from build123d import *

# Parameters (mm, degrees)
F1_DEPTH    = 2.6
F0_W        = 3
F0_H        = 23.3
F0_W_2      = 4.4
F0_H_2      = 0.5
F0_W_3      = 3.9
F2_DEPTH    = 6.1
F3_T1_DEPTH = 6
F3_T3_DEPTH = 5.6650635095
F4_W        = 23
F4_H        = 2
F4_H_2      = 1.9
F5_DEPTH    = 2


# Not quite as in the source:
# - a fillet or chamfer that OpenCascade refuses, or shapes differently, is made with other operations: its cross-section is extruded or revolved along the edge and cut away or added


with BuildPart() as f1:
    # F0 (on Top) → F1 (new body)
    with BuildSketch(Plane.XY):
        Polygon((20, 0), (6.6, 0), (6.6, -5.35), (6.6, -5.85), (2.7, -5.85), (2.7, -5.35), (0, -5.35), (0, -21.3), (2.7, -21.3), (2.7, -20.8), (7.1, -20.8), (7.1, -21.3), (7.1, -23.3), (20, -23.3), align=None)
    extrude(amount=F1_DEPTH)

    # F0 (on Top) → F2 (join)
    with BuildSketch(Plane.XY):
        with Locations((21.5, -11.65)):
            Rectangle(F0_W, F0_H)
        Polygon((2.7, -21.3), (0, -21.3), (0, -23.3), (7.1, -23.3), (7.1, -21.3), align=None)
        Polygon((6.6, 0), (0, 0), (0, -5.35), (2.7, -5.35), (6.6, -5.35), align=None)
        with Locations((4.9, -21.05)):
            Rectangle(F0_W_2, F0_H_2)
        with Locations((4.65, -5.6)):
            Rectangle(F0_W_3, F0_H_2)
    extrude(amount=F2_DEPTH)

    # F3: fillet of radius 1 on 4 edges, made by hand

    # F3_s2 → F3_t1 (cut)
    with BuildSketch(Plane.XY.offset(2.6)):
        with BuildLine():
            ThreePointArc((7.1, -21.8), (6.8071067812, -21.0928932188), (6.1, -20.8))
            Line((6.1, -20.8), (7.1, -20.8))
            Line((7.1, -20.8), (7.1, -21.8))
        make_face()
        with BuildLine():
            ThreePointArc((5.6, -5.85), (6.3071067812, -5.5571067812), (6.6, -4.85))
            Line((6.6, -4.85), (6.6, -5.85))
            Line((6.6, -5.85), (5.6, -5.85))
        make_face()
    extrude(amount=F3_T1_DEPTH, mode=Mode.SUBTRACT)

    # F3_s4 → F3_t3 (cut)
    with BuildSketch(Plane.XY.offset(2.6)):
        with BuildLine():
            ThreePointArc((3.5660254038, -20.8), (3.0660254038, -20.9339745962), (2.7, -21.3))
            Line((2.7, -21.3), (2.7, -20.8))
            Line((2.7, -20.8), (3.5660254038, -20.8))
        make_face()
        with BuildLine():
            ThreePointArc((2.7, -5.35), (3.0660254038, -5.7160254038), (3.5660254038, -5.85))
            Line((3.5660254038, -5.85), (2.7, -5.85))
            Line((2.7, -5.85), (2.7, -5.35))
        make_face()
    extrude(amount=F3_T3_DEPTH, mode=Mode.SUBTRACT)

    # F4 (on Top) → F5 (join)
    with BuildSketch(Plane.XY):
        with Locations((11.5, -22.3)):
            Rectangle(F4_W, F4_H)
        with Locations((11.5, -0.95)):
            Rectangle(F4_W, F4_H_2)
    extrude(amount=-F5_DEPTH)


solid = f1.part
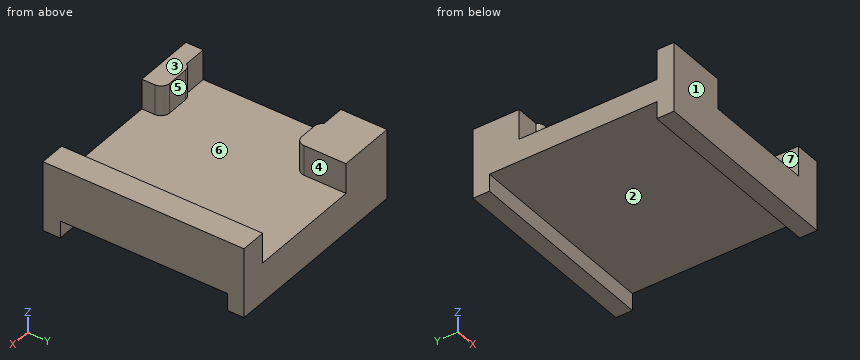
Design review of the part built by this model. Coordinates are the model's own, in mm. Face numbers are marked on the shaded views. A direction names the side the tool comes from. Round coordinates to 2 decimals unless told otherwise and drop trailing zeros. Order: outer loops, then holes, each group sorted by start corner. A loop starts at its lowest first (then second) coordinate and runs counter-clockwise, first axis right, second up.
1) Consider section C-C (y = -3.5). State the section outline as (x, z) points, plus the area to 3 significant figures.
The answers:
outline: (0, 0) - (23, 0) - (23, 6.1) - (20, 6.1) - (20, 2.6) - (6.6, 2.6) - (6.6, 6.1) - (0, 6.1) - close
area: 93.4 mm2
2) Draft analysis for pull direction Y (two halves, no side actions). For the marked faces 1, 2 and 3, state which applies: released by +Y, released by -Y, zero draft, split by the parting line, or undercut.
The answers:
face 1: released by -Y
face 2: undercut
face 3: zero draft
3) For L1, parallel to Y at x = 1.5, z = 3.5; L2, parallel to Y at x = 3, z = -0.25; L3, parallel to Z at x = 14.25, y = -6.25, list the stretches that pass through material, from the lowest coordinate up.
The answers:
L1: y = -23.3 to -21.3, -5.35 to 0
L2: y = -23.3 to -21.3, -1.9 to 0
L3: z = 0 to 2.6
4) Clearance check with flat-ended pins moving along their axes: pin 1 Ø12 at (x, y) = (3.5, -13) entering from -Z; pin 2 Ø1 at (y, z) = (-11, 5) entering from -X; pin 3 Ø1.3 at (x, z) = (4.5, 4) entering from +Y; pin 4 Ø3 at (x, y) = (3.5, -10.5) entering from +Z. State where each tip first meets the part, or that it passes through.
The answers:
pin 1: stops at z = 0
pin 2: stops at x = 20
pin 3: stops at y = 0
pin 4: stops at z = 2.6
5) Machinability: for the marked faces 4, 5, 6 and 7, which of the approach directions +Z, -Z, +X, -X, +Y, -Y give a long, thin tool a straight path to every point of the face, cutting with its end or side? Answer none if there is none.
The answers:
face 4: +Z, +Y
face 5: +Z, -X
face 6: +Z
face 7: +Z, +Y, -Y
6) Consider section D-D (y = -17.5). State the section outline as (x, z) points.
The answers:
outline: (0, 0) - (23, 0) - (23, 6.1) - (20, 6.1) - (20, 2.6) - (0, 2.6) - close
7) Consider section A-A (z = 5.5). State the section outline as (x, y) points, plus the area to 3 significant figures.
The answers:
outline: (0, -23.3) - (7.1, -23.3) - (7.1, -21.8) arc R1 ccw to (6.1, -20.8) - (3.57, -20.8) arc R1 ccw to (2.7, -21.3) - (0, -21.3) - close; (0, -5.35) - (2.7, -5.35) arc R1 ccw to (3.57, -5.85) - (5.6, -5.85) arc R1 ccw to (6.6, -4.85) - (6.6, 0) - (0, 0) - close; (20, -23.3) - (23, -23.3) - (23, 0) - (20, 0) - close
area: 123 mm2
8) Consider section B-B (x = 5.25). State the section outline as (y, z) points, plus the area to 3 significant figures.
The answers:
outline: (-23.3, -2) - (-21.3, -2) - (-21.3, 0) - (-1.9, 0) - (-1.9, -2) - (0, -2) - (0, 6.1) - (-5.85, 6.1) - (-5.85, 2.6) - (-20.8, 2.6) - (-20.8, 6.1) - (-23.3, 6.1) - close
area: 97.6 mm2
